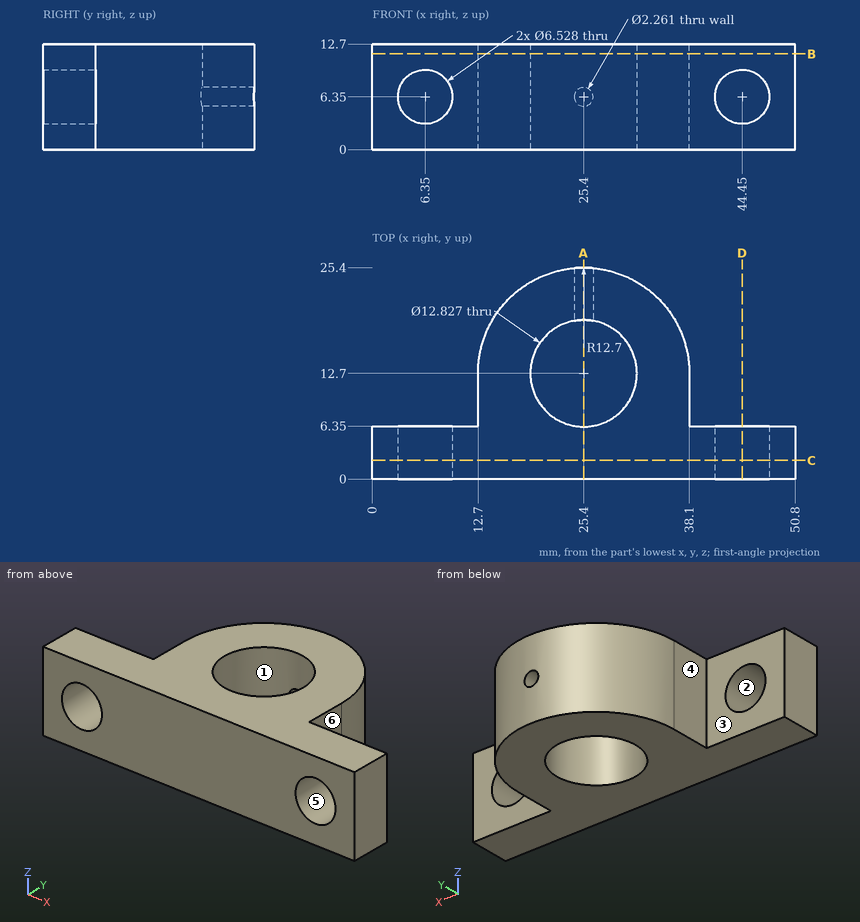
Drawing for the job (mm, zero at the part's lowest x, y, z). A direction names the side the tool comes from. Give positions to 0.01 mm unless a question says otherwise; leave off trailing zeros. Loops run counter-clockwise (first coordinate to the right, second up) from the corner with the lowest first, then second, coordinate; pieces in that order, holes last.
Item 1: Drill centre lines: line 1 along X through (y, z) = (1.75, 3.75) (1 decimal); line 2 along Y through (x, z) = (25.4, 6.5); line 3 along Z through (x, y) = (6.35, 5.25). Where is each one in solid material? Low to high.
Check values:
line 1: x = 0 to 4.4, 8.3 to 42.5, 46.4 to 50.8
line 2: y = 0 to 6.29
line 3: z = 0 to 3.09, 9.61 to 12.7
Item 2: Slice it at A-A (x = 25.4). Write the cut outline in (y, z).
Check values:
outline: (0, 0) - (6.29, 0) - (6.29, 12.7) - (0, 12.7) - close; (19.11, 0) - (25.4, 0) - (25.4, 5.22) - (19.11, 5.22) - close; (19.11, 7.48) - (25.4, 7.48) - (25.4, 12.7) - (19.11, 12.7) - close
Item 3: Slice it at D-D (x = 44.45). Write the cut outline in (y, z).
Check values:
outline: (0, 0) - (6.35, 0) - (6.35, 3.09) - (0, 3.09) - close; (0, 9.61) - (6.35, 9.61) - (6.35, 12.7) - (0, 12.7) - close
Item 4: Slice it at C-C (y = 2.25). Write the cut outline in (x, z).
Check values:
outline: (0, 0) - (50.8, 0) - (50.8, 12.7) - (0, 12.7) - close; hole circle Ø6.53 at (6.35, 6.35); hole circle Ø6.53 at (44.45, 6.35)
Item 5: Mould opens along Y. For the marked faces 1, 2 and 3 say: +Y half, -Y half, draft (parallel to the pull), parting line (faces both ways), or undercut.
Check values:
face 1: undercut
face 2: draft
face 3: +Y half
Item 6: Which spindle directions (+Z, -Z, +X, -X, +Y, -Y) get a long thin tool onto all of the face, cutting with end or side? Do the marked faces 4, 5 and 6. Say none if no direction does.
Check values:
face 4: +Z, -Z, -X, +Y
face 5: +Y, -Y
face 6: +Z, -Z, +X, +Y
Item 7: Slice it at B-B (z = 11.5). Write the cut outline in (x, y), plus the area to 3 significant figures.
Check values:
outline: (0, 0) - (50.8, 0) - (50.8, 6.35) - (38.1, 6.35) - (38.1, 12.7) arc R12.7 ccw to (12.7, 12.7) - (12.7, 6.35) - (0, 6.35) - close; hole circle Ø12.83 at (25.4, 12.7)
area: 608 mm2
Item 8: Drop flat-ended pins along their axis: P1, Ø6, axis at x = 44.45, z = 6.35, coming from the -Y side; P2, Ø4, axis at x = 33.5, z = 3.5, coming from the +Y side; P3, Ø3, axis at x = 20, z = 5, coming from the +Y side; P4, Ø4, axis at x = 3.5, z = 7, coming from the +Y side. Give the stop position or say it passes through.
Check values:
P1: passes through
P2: stops at y = 23.84
P3: stops at y = 24.79
P4: stops at y = 6.35
